```python
from build123d import *

# Parameters (mm, degrees)
SKETCH1_W           = 127
SKETCH1_H           = 25.4
BOSS_EXTRUDE1_DEPTH = 88.9
BOSS_EXTRUDE2_DEPTH = 25.4
BOSS_EXTRUDE3_DEPTH = 63.5


with BuildPart() as part:
    # Sketch1 → Boss-Extrude1 (new body)
    with BuildSketch(Plane.XY):
        with Locations((63.5, 12.7)):
            Rectangle(SKETCH1_W, SKETCH1_H)
    extrude(amount=BOSS_EXTRUDE1_DEPTH)

    # Sketch1_3 → Boss-Extrude2 (add)
    with BuildSketch(Plane.XY):
        with BuildLine():
            Line((0, 101.6), (0, 25.4))
            Line((0, 25.4), (63.5, 25.4))
            Line((63.5, 25.4), (63.5, 101.6))
            ThreePointArc((63.5, 101.6), (31.75, 69.85), (0, 101.6))
        make_face()
    extrude(amount=BOSS_EXTRUDE2_DEPTH)

    # Sketch1_4 → Boss-Extrude3 (add)
    with BuildSketch(Plane.XY):
        with BuildLine():
            ThreePointArc((63.5, 101.6), (31.75, 133.35), (0, 101.6))
            Line((0, 101.6), (15.875, 101.6))
            ThreePointArc((15.875, 101.6), (31.75, 117.475), (47.625, 101.6))
            Line((47.625, 101.6), (63.5, 101.6))
        make_face()
        with BuildLine():
            Line((15.875, 101.6), (0, 101.6))
            ThreePointArc((0, 101.6), (31.75, 69.85), (63.5, 101.6))
            Line((63.5, 101.6), (47.625, 101.6))
            ThreePointArc((47.625, 101.6), (31.75, 85.725), (15.875, 101.6))
        make_face()
    extrude(amount=BOSS_EXTRUDE3_DEPTH)


solid = part.part
```
Here's how the part is built. I have some questions about the finished solid (model axes, mm). A direction names the side the tool comes from. Give positions to 0.01 mm unless a question says otherwise; leave off trailing zeros. Loops run counter-clockwise (first coordinate to the right, second up) from the corner with the lowest first, then second, coordinate; pieces in that order, holes last. Notation, with made-up numbers: M 7.5,-3.5 L 61.5,-3.5 A23 ccw 61.5,11.5 Z; hole C 73.5,-7.5 d3. An arc over 180 degrees is marked long. Return JSON: item names as keys, results as strings.
Item 1: I'm going to push flat-ended pins straight in: pin 1 Ø6 at (x, z) = (96.5, 54.5) entering from +Y; pin 2 Ø4 at (y, z) = (88.5, 56.5) entering from -X; pin 3 Ø1 at (x, z) = (55, 21.5) entering from +Y. Where does each tip first touch, or does it pass through?
A:
{"pin 1": "stops at y = 25.4", "pin 2": "stops at x = 2", "pin 3": "stops at y = 123.75"}
Item 2: Imagine slicing it at C-C on x = 54.5. List the corners of the cut face in (y, z) for me.
A:
{"outline": "M 0,0 L 123.75,0 L 123.75,63.5 L 79.45,63.5 L 79.45,25.4 L 25.4,25.4 L 25.4,88.9 L 0,88.9 Z"}
Item 3: Imagine slicing it at D-D on z = 69.5. List the corners of the cut face in (x, y) for me, then the cut area to 3 significant figures.
A:
{"outline": "M 0,0 L 127,0 L 127,25.4 L 0,25.4 Z", "area": "3,230 mm^2"}
Item 4: Thinking about a two-plate mould opening in Y: for faces 1 (the cylindrical face through (28.309, 117.097, 31.306)), 2 (the flat face through (63, 0, 44)), 3 (the flat face through (38.4, 116.2, 63.5)), which applies, released by +Y, released by -Y, zero draft, split by the parting line, or undercut?
A:
{"face 1": "undercut", "face 2": "released by -Y", "face 3": "zero draft"}
Item 5: Imagine slicing it at B-B on x = 31.75. List the corners of the cut face in (y, z) for me (3 decimals).
A:
{"outline": "M 0,0 L 85.725,0 L 85.725,63.5 L 69.85,63.5 L 69.85,25.4 L 25.4,25.4 L 25.4,88.9 L 0,88.9 Z; M 117.475,0 L 133.35,0 L 133.35,63.5 L 117.475,63.5 Z"}
Item 6: Please list where these lines run through material, in increasing order: line 1 (Y direction, x = 31, z = 29); line 2 (X direction, y = 101.6, z = 44) (3 decimals); line 3 (Z direction, x = 60, y = 37).
A:
{"line 1": "y = 0 to 25.4, 69.86 to 85.74, 117.46 to 133.34", "line 2": "x = 0 to 15.875, 47.625 to 63.5", "line 3": "z = 0 to 25.4"}
Item 7: On a 3-axis mill with a long thin cutter (end or side, diameter ignored), from which of +Z, -Z, +X, -X, +Y, -Y can I reach the whole of each face in a straight line? I mean faces 4 (the cylindrical face through (17.1, 129.77, 38.36)), 5 (the flat face through (63.5, 63, 13)), 6 (the flat face through (63, 25.4, 54)). Say none if no direction works.
A:
{"face 4": "+Z", "face 5": "+Z, -Z, +X, +Y", "face 6": "+Z, +X"}
Item 8: Imagine slicing it at A-A on z = 44. List the corners of the cut face in (x, y) for me (3 decimals), then the cut area to 3 significant figures.
A:
{"outline": "M 0,0 L 127,0 L 127,25.4 L 0,25.4 Z; C 31.75,101.6 d63.5; hole C 31.75,101.6 d31.75", "area": "5,600 mm^2"}
